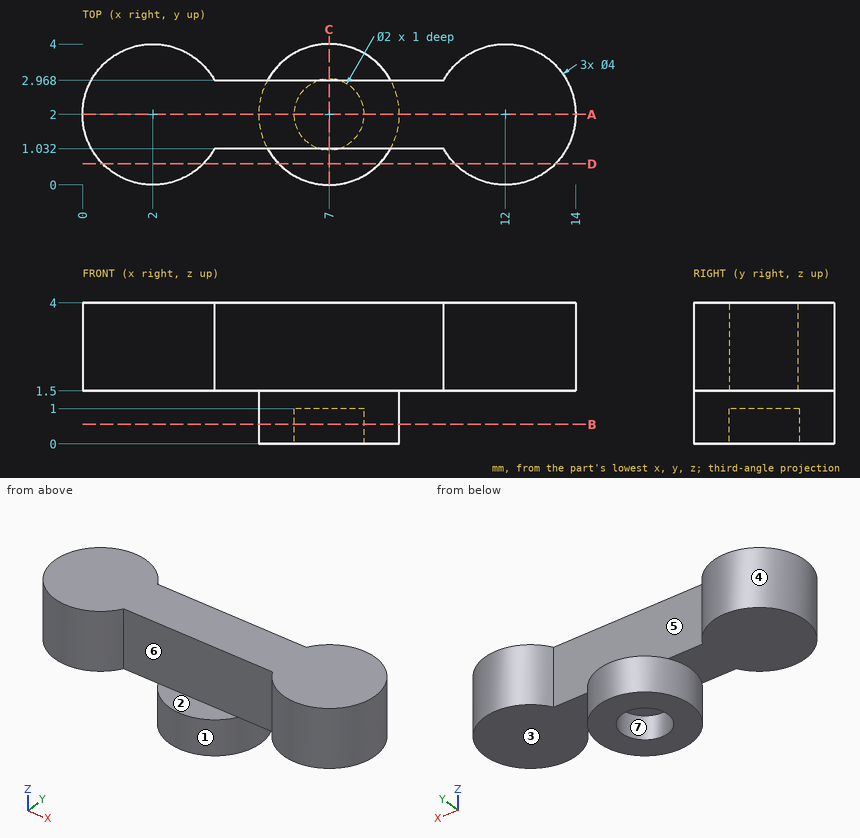
Study the drawing (mm; zero at the part's minimum x, y, z) and answer. A direction names the side the tool comes from. Coordinates: 2 decimals unless noted, no trailing zeros. Loops run counter-clockwise (first coordinate to the right, second up) from the corner with the lowest first, then second, coordinate; pieces in that order, holes last. Notation, with made-up numbers: (18, 81) -> (69, 81) arc R24 ccw to (69, 111) -> close; hole circle Ø1 at (-22.5, -40). An arc over 180 degrees is marked (long way). Answer in a Markdown table with one row per item. Add a question column.
1. Consider line 1 (Y direction, x = 7, z = 0.6); line 2 (Z direction, x = 11.25, y = 0.7); line 3 (X direction, y = 3.2, z = 2.95). Determine where each line is inside the solid, lowest interval first. Write a range as [from, to].
2. For the marked faces 4, 5, 6 and 7, determine the directions among +Z, -Z, +X, -X, +Y, -Y from which every point of the face is accessible in a straight line to the end or side of a thin tool.
3. The part is cut by section B-B, the plane z = 0.55. Write down the section's boundary in (x, y).
4. The part is cut by section A-A, the plane y = 2. Write down the section's boundary in (x, z), then the cut area to 3 significant figures.
5. Determine the mould class of the marked faces 1, 2 and 3 for opening direction X: +X half, -X half, draft (parallel to the pull), parting line (faces both ways), or undercut.
6. The part is cut by section D-D, the plane y = 0.6. Write down the section's boundary in (x, z).
7. The part is cut by section C-C, the plane x = 7. Write down the section's boundary in (y, z).
8. Flat-ended cylindrical pins translate along their axes: P1, Ø1.2, axis at x = 10.5, y = 1.5, coming from the -Z side; P2, Ø2, axis at x = 5.5, z = 2, coming from the +Y side; P3, Ø1.5, axis at y = 3, z = 1.5, coming from the -X side. Find the tip coordinate at first contact, or state that the pin passes through.
Answer below:
| question | item | result |
|---|---|---|
| 1 | line 1 | [0, 1], [3, 4] |
| 1 | line 2 | [1.5, 4] |
| 1 | line 3 | [0.4, 3.6], [10.4, 13.6] |
| 2 | face 4 | +Z, -Z |
| 2 | face 5 | +Z, +Y |
| 2 | face 6 | +Z, -Y |
| 2 | face 7 | -Z |
| 3 | outline | circle Ø4 at (7, 2); hole circle Ø2 at (7, 2) |
| 4 | outline | (0, 1.5) -> (5, 1.5) -> (5, 0) -> (6, 0) -> (6, 1) -> (8, 1) -> (8, 0) -> (9, 0) -> (9, 1.5) -> (14, 1.5) -> (14, 4) -> (0, 4) -> close |
| 4 | area | 39.0 mm2 |
| 5 | face 1 | parting line |
| 5 | face 2 | undercut |
| 5 | face 3 | draft |
| 6 | outline | (0.57, 1.5) -> (3.43, 1.5) -> (3.43, 4) -> (0.57, 4) -> close; (5.57, 0) -> (8.43, 0) -> (8.43, 1.5) -> (5.57, 1.5) -> close; (10.57, 1.5) -> (13.43, 1.5) -> (13.43, 4) -> (10.57, 4) -> close |
| 7 | outline | (0, 0) -> (1, 0) -> (1, 1) -> (3, 1) -> (3, 0) -> (4, 0) -> (4, 1.5) -> (2.97, 1.5) -> (2.97, 4) -> (1.03, 4) -> (1.03, 1.5) -> (0, 1.5) -> close |
| 8 | P1 | z = 1.5 |
| 8 | P2 | y = 3.9 |
| 8 | P3 | x = 0.02 |
